Verification items for the finished model (mm, model axes). Face numbers are marked on the shaded views. A direction names the side the tool comes from. Give positions to 0.01 mm unless a question says otherwise; leave off trailing zeros. Order: outer loops, then holes, each group sorted by start corner. A loop starts at its lowest first (then second) coordinate and runs counter-clockwise, first axis right, second up. Notation, with made-up numbers: (70.5, 59.25) -> (100.5, 59.25) arc R8 ccw to (100.5, 68.25) -> close; hole circle Ø10 at (73.25, 56.25). An arc over 180 degrees is marked (long way). One line per question, with ' | ' between items. Start each with the question number.
Q1. Section check B-B on x = 0. Record the cut outline in (y, z), plus the area to 3 significant figures.
Q2. Access from +Z, -Z, +X, -X, +Y, -Y to the whole of each face (thin tool, end or side, straight path). Record for the marked faces 4 and 5.
Q3. Go/stop test with flat-tipped pins: pin 1 (6 mm diameter, centred on y = 14, z = -5.5, fed in from -X); pin 2 (8 mm diameter, centred on y = 5, z = -9.5, fed in from +X). Record where each tip stops, or that it passes through.
Q4. Section check C-C on y = -0.5. Record the cut outline in (x, z), plus the area to 3 significant figures.
Q5. Material ranges on probe 1 along Z at (x, y) = (0, 12); probe 2 along Z at (x, y) = (0, 9.5); probe 3 along X at (y, z) = (5.5, 3), recorded low to high. Write a range as [from, to].
Q6. Section check A-A on z = 0. Record the cut outline in (x, y), plus the area to 3 significant figures.
Q7. Mould release check, pull along Z, two halves, no side actions. Record for the marked faces 1, 2 and 3: released by +Z, released by -Z, zero draft, split by the parting line, or undercut.
Q8. Section check D-D on x = -7. Record the cut outline in (y, z), plus the area to 3 significant figures.
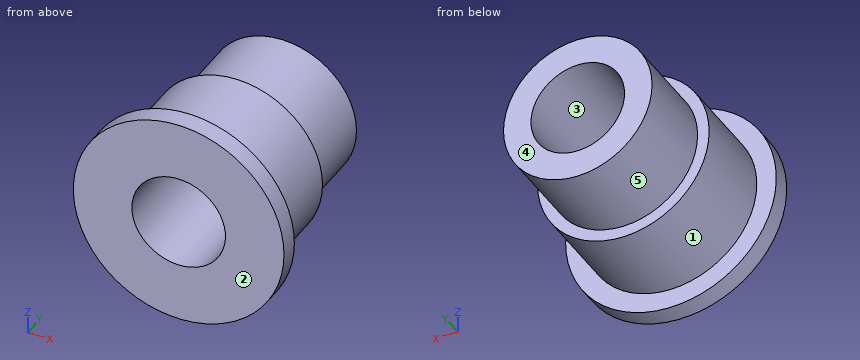
from build123d import *

# Parameters (mm, degrees)
F0_R     = 13.5
F0_R_2   = 11.985483
F1_DEPTH = 2.5
F2_R     = 11
F3_DEPTH = 11.5
F4_R     = 9.52
F5_DEPTH = 11
F6_R     = 6
F7_DEPTH = 25


with BuildPart() as f1:
    # F0 (on Front) → F1 (new body)
    with BuildSketch(Plane.XZ):
        Circle(F0_R)
        Circle(F0_R_2, mode=Mode.SUBTRACT)
        Circle(F0_R_2)
    extrude(amount=F1_DEPTH)

    # F2 (on face) → F3 (join)
    with BuildSketch(Plane(origin=(0, 0, 0), x_dir=(-1, 0, 0), z_dir=(0, 1, 0))):
        Circle(F2_R)
    extrude(amount=F3_DEPTH)

    # F4 (on face) → F5 (join)
    with BuildSketch(Plane(origin=(0, 11.5, 0), x_dir=(-1, 0, 0), z_dir=(0, 1, 0))):
        Circle(F4_R)
    extrude(amount=F5_DEPTH)

    # F6 (on face) → F7 (cut)
    with BuildSketch(Plane(origin=(0, 22.5, 0), x_dir=(-1, 0, 0), z_dir=(0, 1, 0))):
        Circle(F6_R)
    extrude(amount=-F7_DEPTH, mode=Mode.SUBTRACT)


solid = f1.part
Filled in:
1) outline: (-2.5, -13.5) -> (0, -13.5) -> (0, -11) -> (11.5, -11) -> (11.5, -9.52) -> (22.5, -9.52) -> (22.5, -6) -> (-2.5, -6) -> close; (-2.5, 6) -> (22.5, 6) -> (22.5, 9.52) -> (11.5, 9.52) -> (11.5, 11) -> (0, 11) -> (0, 13.5) -> (-2.5, 13.5) -> close | area: 230 mm²
2) face 4: +Z, -Z, +X, -X, +Y | face 5: +Y
3) pin 1: x = -10.31 | pin 2: x = 9.53
4) outline: circle Ø27 at (0, 0); hole circle Ø12 at (0, 0) | area: 459 mm²
5) probe 1: [-9.52, -6], [6, 9.52] | probe 2: [-11, -6], [6, 11] | probe 3: [-10.58, -5.2], [5.2, 10.58]
6) outline: (-13.5, -2.5) -> (-6, -2.5) -> (-6, 22.5) -> (-9.52, 22.5) -> (-9.52, 11.5) -> (-11, 11.5) -> (-11, 0) -> (-13.5, 0) -> close; (6, -2.5) -> (13.5, -2.5) -> (13.5, 0) -> (11, 0) -> (11, 11.5) -> (9.52, 11.5) -> (9.52, 22.5) -> (6, 22.5) -> close | area: 230 mm²
7) face 1: split by the parting line | face 2: zero draft | face 3: undercut
8) outline: (-2.5, -11.54) -> (0, -11.54) -> (0, -8.49) -> (11.5, -8.49) -> (11.5, -6.45) -> (22.5, -6.45) -> (22.5, 6.45) -> (11.5, 6.45) -> (11.5, 8.49) -> (0, 8.49) -> (0, 11.54) -> (-2.5, 11.54) -> close | area: 395 mm²
